CAD build for the part. Positions are in the model's coordinates, mm. Face numbers are marked on the shaded views. A direction names the side the tool comes from. Round coordinates to 2 decimals unless told otherwise and drop trailing zeros. Loops run counter-clockwise (first coordinate to the right, second up) from the corner with the lowest first, then second, coordinate; pieces in that order, holes last. Notation, with made-up numbers: M -12.75,4 L 43.25,4 A24 ccw 43.25,15 Z; hole C 85,84 d4. An arc over 180 degrees is marked long. One line per item, written item: value. Start each with the question number.
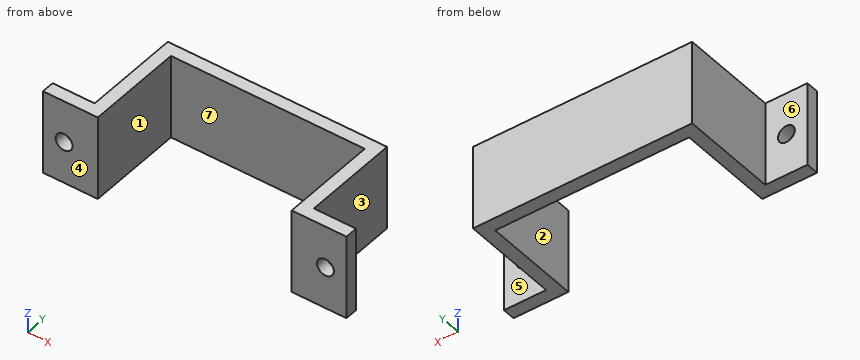
from build123d import *

# Parameters (mm, degrees)
BOSS_EXTRUDE1_DEPTH     = 10
CUT_EXTRUDE1_DEPTH      = 24.58495283
CUT_EXTRUDE1_DEPTH_BACK = 24.58495283
SKETCH2_R               = 1


with BuildPart() as part:
    # Sketch1 → Boss-Extrude1 (new body)
    with BuildSketch(Plane.XY):
        Polygon((-11.5, 0), (-11.5, 10), (11.5, 10), (11.5, 0), (11.5, -1.5), (18, -1.5), (18, 0), (13, 0), (13, 11.5), (-13, 11.5), (-13, 0), (-18, 0), (-18, -1.5), (-11.5, -1.5), align=None)
    extrude(amount=BOSS_EXTRUDE1_DEPTH)

    # Sketch2 → Cut-Extrude1 (cut, two sides: drawn at the far end of the back side and taken through both)
    with BuildSketch(Plane(origin=(0, 0, 0), x_dir=(1, 0, 0), z_dir=(0, 1, 0)).offset(-CUT_EXTRUDE1_DEPTH_BACK)):
        with Locations(Location((-15.5, -5, 0), (0, 0, 180))):
            Circle(SKETCH2_R)
        with Locations((15.5, -5)):
            Circle(SKETCH2_R)
    extrude(amount=CUT_EXTRUDE1_DEPTH + CUT_EXTRUDE1_DEPTH_BACK, mode=Mode.SUBTRACT)


solid = part.part
(1) Slice it at D-D, the plane y = 7.75. List the corners of the cut face in (x, z), and give its area (3 significant figures).
(2) Slice it at A-A, the plane y = -0.5. List the corners of the cut face in (x, z).
(3) Which spindle directions (+Z, -Z, +X, -X, +Y, -Y) get a long thin tool onto all of the face, cutting with end or side? Do the marked faces 5, 6 and 7. Say none if no direction does.
(4) Mould opens along X. For the marked faces 1, 2, 3 and 4 say: pulls with the +X half, pulls with the -X half, needs draft (parallel to the pull), parting line crosses it, or undercut.
(5) Slice it at C-C, the plane z = 5. List the corners of the cut face in (x, y), and give its area (3 significant figures).
(6) Flat gauge pins, fed straight in: P1, Ø1, axis at y = 1, z = 4.5, coming from the +X side; P2, Ø5, axis at y = 6, z = 4.5, coming from the -X side; P3, Ø5.5, axis at x = 16, z = 3.5, coming from the +Y side; P4, Ø1.8, axis at x = -15.5, z = 5, coming from the -Y side (3 decimals). Where does each tip first touch, or does it go through?
(7) Slice it at B-B, the plane x = 15.5. List the corners of the cut face in (y, z).
(8) Probe L1, parallel to X at y = 9.5, z = 7; L2, parallel to Z at x = 15.5, y = -0.85; L3, parallel to Y at x = -5.5, z = 2.5. List the from-to ranges inside material, lowest first.
Check result:
1. outline: M -13,0 L -11.5,0 L -11.5,10 L -13,10 Z; M 11.5,0 L 13,0 L 13,10 L 11.5,10 Z
1. area: 30.0 mm^2
2. outline: M -18,0 L -11.5,0 L -11.5,10 L -18,10 Z; M 11.5,0 L 18,0 L 18,10 L 11.5,10 Z; hole C -15.5,5 d2; hole C 15.5,5 d2
3. face 5: +Z, -Z, +X, +Y
3. face 6: +Z, -Z, -X, +Y
3. face 7: +Z, -Z, -Y
4. face 1: undercut
4. face 2: undercut
4. face 3: pulls with the +X half
4. face 4: needs draft
5. outline: M -18,-1.5 L -16.5,-1.5 L -16.5,0 L -18,0 Z; M -14.5,-1.5 L -11.5,-1.5 L -11.5,10 L 11.5,10 L 11.5,-1.5 L 14.5,-1.5 L 14.5,0 L 13,0 L 13,11.5 L -13,11.5 L -13,0 L -14.5,0 Z; M 16.5,-1.5 L 18,-1.5 L 18,0 L 16.5,0 Z
5. area: 82.5 mm^2
6. P1: stops at x = 13
6. P2: stops at x = -13
6. P3: stops at y = 0
6. P4: passes through
7. outline: M -1.5,0 L 0,0 L 0,4 L -1.5,4 Z; M -1.5,6 L 0,6 L 0,10 L -1.5,10 Z
8. L1: x = -13 to -11.5, 11.5 to 13
8. L2: z = 0 to 4, 6 to 10
8. L3: y = 10 to 11.5
